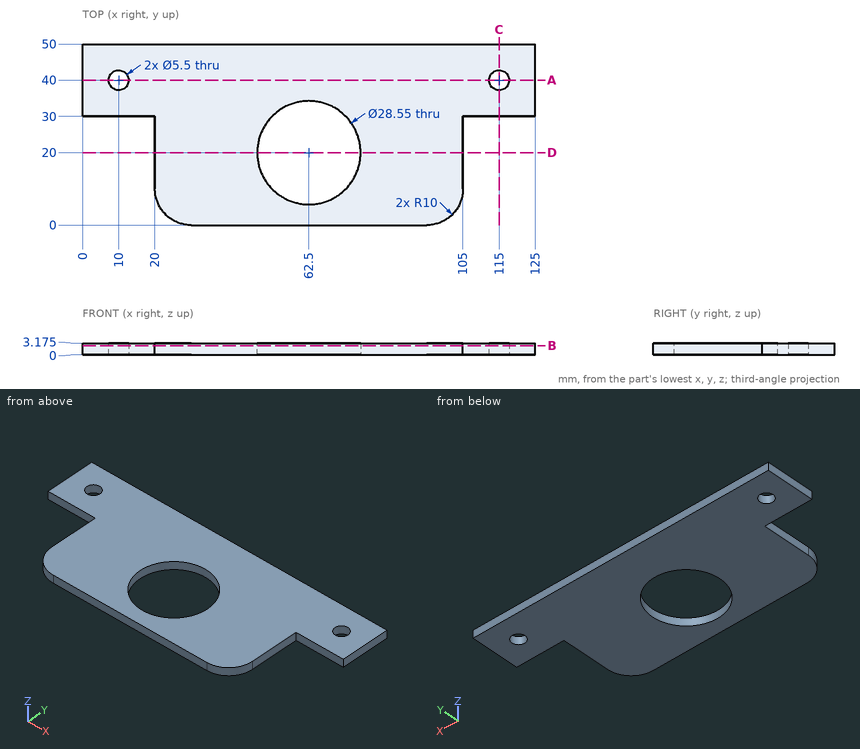
Here's the drawing with two shaded views (mm, measured from the low corner). I have some questions. Coordinates: 2 decimals unless noted, no trailing zeros. Loops run counter-clockwise (first coordinate to the right, second up) from the corner with the lowest first, then second, coordinate; pieces in that order, holes last.
Item 1: I'm going to push flat-ended pins straight in: pin 1 (1 mm diameter, centred on x = 73.5, y = 11.5, fed in from -Z); pin 2 (17 mm diameter, centred on x = 62.5, y = 20, fed in from +Z); pin 3 (1 mm diameter, centred on x = 114, z = 2.5, fed in from -Y); pin 4 (1.5 mm diameter, centred on y = 25, z = 2, fed in from -X). Where does each tip first touch, or does it pass through?
Answers below:
pin 1: stops at z = 0
pin 2: passes through
pin 3: stops at y = 30
pin 4: stops at x = 20
Item 2: Suppose I cut it at D-D (y = 20). Please give me the cut outline in (x, z) (3 decimals).
Answers below:
outline: (20, 0) - (48.225, 0) - (48.225, 3.175) - (20, 3.175) - close; (76.775, 0) - (105, 0) - (105, 3.175) - (76.775, 3.175) - close
Item 3: Please list where these lines run through material, in increasing order: L1, parallel to Y at x = 10, z = 1.4; L2, parallel to Y at x = 62.5, z = 1.2 (3 decimals); L3, parallel to X at y = 27, z = 1.5.
Answers below:
L1: y = 30 to 37.25, 42.75 to 50
L2: y = 0 to 5.725, 34.275 to 50
L3: x = 20 to 50.06, 74.94 to 105
Item 4: Suppose I cut it at C-C (x = 115). Please give me the cut outline in (y, z) (3 decimals).
Answers below:
outline: (30, 0) - (37.25, 0) - (37.25, 3.175) - (30, 3.175) - close; (42.75, 0) - (50, 0) - (50, 3.175) - (42.75, 3.175) - close
Item 5: Suppose I cut it at B-B (z = 2.5). Please give me the cut outline in (x, y) (3 decimals).
Answers below:
outline: (0, 30) - (20, 30) - (20, 10) arc R10 ccw to (30, 0) - (95, 0) arc R10 ccw to (105, 10) - (105, 30) - (125, 30) - (125, 50) - (0, 50) - close; hole circle Ø5.5 at (10, 40); hole circle Ø28.55 at (62.5, 20); hole circle Ø5.5 at (115, 40)
Item 6: Suppose I cut it at A-A (y = 40). Please give me the cut outline in (x, z) (3 decimals).
Answers below:
outline: (0, 0) - (7.25, 0) - (7.25, 3.175) - (0, 3.175) - close; (12.75, 0) - (112.25, 0) - (112.25, 3.175) - (12.75, 3.175) - close; (117.75, 0) - (125, 0) - (125, 3.175) - (117.75, 3.175) - close
